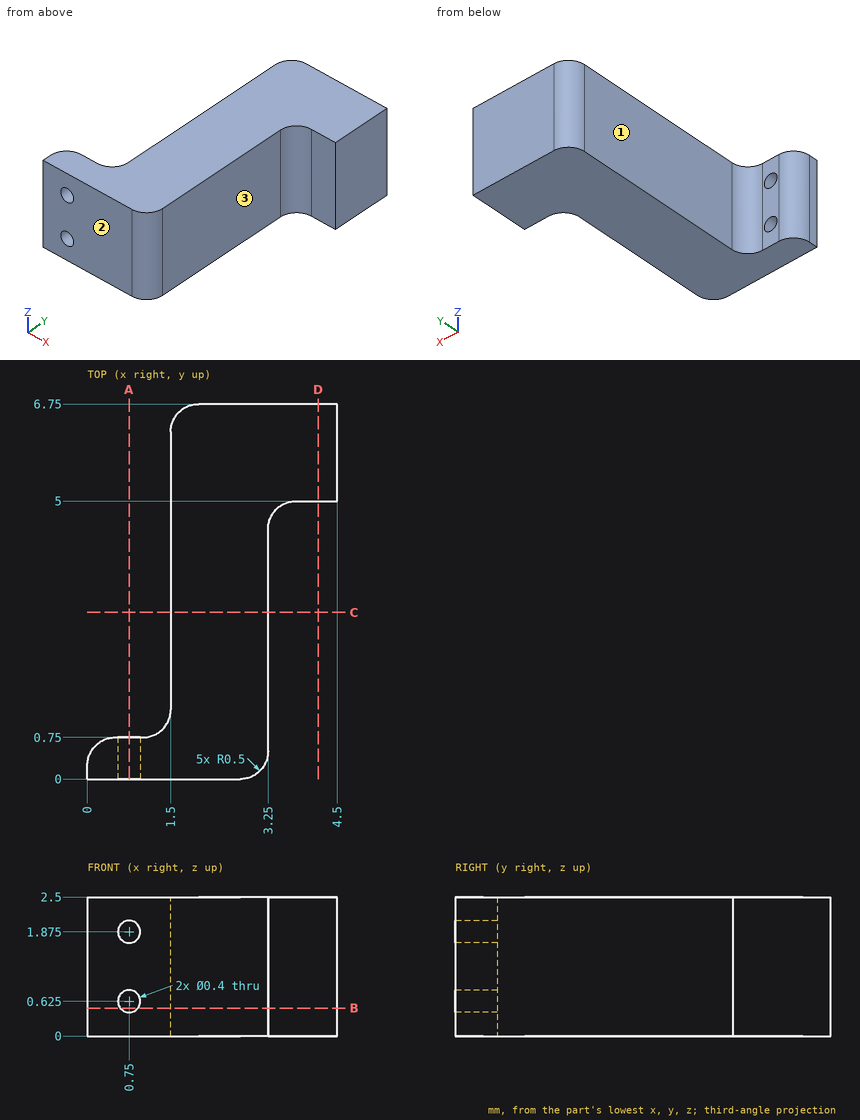
Design review of the part shown in the three views and the two pictorial views. Dimensions are in mm from the part's minimum x, y and z. A direction names the side the tool comes from. Coordinates: 2 decimals unless noted, no trailing zeros. Order: outer loops, then holes, each group sorted by start corner. A loop starts at its lowest first (then second) coordinate and runs counter-clockwise, first axis right, second up.
Item 1: Take a section at C-C, the plane y = 3. Write out the cut boundary in (x, z), then the cut area to 4 significant figures.
Item 2: Take a section at D-D, the plane x = 4.15. Write out the cut boundary in (y, z), then the cut area to 4 significant figures.
Item 3: For the marked faces 1, 2 and 3, list the 3-axis set-ups (+Z, -Z, +X, -X, +Y, -Y) from which the entire face can be reached by the end or side of a thin tool; tool diameter is ignored.
Item 4: For line 1 (Z direction, x = 0.75, y = 0.2) (3 decimals); line 2 (X direction, y = 4.25, z = 1.55); line 3 (X direction, y = 5.25, z = 1.8), list the stretches that pass through material, from the lowest coordinate up.
Item 5: For pin 1 Ø1.2 at (y, z) = (3.5, 1.5) entering from -X; pin 2 Ø1.2 at (y, z) = (2, 1.5) entering from +X; pin 3 Ø0.8 at (x, z) = (4.5, 1) entering from -Y, all flat-tipped, find the tip position at first contact; note any pin that passes through.
Item 6: Take a section at B-B, the plane z = 0.5. Write out the cut boundary in (x, y).
Item 7: Take a section at A-A, the plane x = 0.75. Write out the cut boundary in (y, z) (3 decimals), then the cut area to 4 significant figures.
The answers:
1. outline: (1.5, 0) - (3.25, 0) - (3.25, 2.5) - (1.5, 2.5) - close
1. area: 4.375 mm2
2. outline: (5, 0) - (6.75, 0) - (6.75, 2.5) - (5, 2.5) - close
2. area: 4.375 mm2
3. face 1: +Z, -Z, -X, +Y
3. face 2: +Z, -Z, +X, -X, -Y
3. face 3: +Z, -Z, +X, -Y
4. line 1: z = 0 to 0.425, 0.825 to 1.675, 2.075 to 2.5
4. line 2: x = 1.5 to 3.25
4. line 3: x = 1.5 to 4.5
5. pin 1: stops at x = 1.5
5. pin 2: stops at x = 3.25
5. pin 3: stops at y = 5
6. outline: (0, 0) - (0.59, 0) - (0.59, 0.75) - (0.5, 0.75) arc R0.5 ccw to (0, 0.25) - close; (0.91, 0) - (2.75, 0) arc R0.5 ccw to (3.25, 0.5) - (3.25, 4.5) arc R0.5 cw to (3.75, 5) - (4.5, 5) - (4.5, 6.75) - (2, 6.75) arc R0.5 ccw to (1.5, 6.25) - (1.5, 1.25) arc R0.5 cw to (1, 0.75) - (0.91, 0.75) - close
7. outline: (0, 0) - (0.75, 0) - (0.75, 0.425) - (0, 0.425) - close; (0, 0.825) - (0.75, 0.825) - (0.75, 1.675) - (0, 1.675) - close; (0, 2.075) - (0.75, 2.075) - (0.75, 2.5) - (0, 2.5) - close
7. area: 1.275 mm2
